Autodesk Fusion 360 part; units mm, degrees
sketch "Sketch1" plane through (0, 0, 0) normal (1, 0, 0) x (0, 1, 0)
  line L0 (0, 0) -> (27, 0)
  line L1 (27, 0) -> (27, 16)
  line L2 (27, 16) -> (0, 16)
  line L3 (0, 16) -> (0, 0)
  line L4 (0, 9.5) -> (6, 9.5) construction
  line L5 (6, 9.5) -> (6, 16) construction
  circle A0 centre (6, 9.5) radius 3
  line L6 (6, 9.5) -> (21, 9.5)
  circle A1 centre (21, 9.5) radius 3
  dimension "d1_4" = 16
  dimension "d2_4" = 27
  dimension "d3_4" = 6
  dimension "d4_4" = 6.5
  dimension "d5_2" = 6
  dimension "d6_1" = 15
  dimension "d7_2" = 6
extrude "Extrude1" add sketch "Sketch1" along normal blind 3 makes body 1
sketch "Sketch2" plane through (0, 0, 0) normal (-1, 0, 0) x (0, -1, 0)
  circle A0 centre (-21, 9.5) radius 3
  circle A1 centre (-6, 9.5) radius 3
  line L0 (0, 0) -> (0, 16)
  line L1 (0, 16) -> (-27, 16)
  line L2 (-27, 16) -> (-27, 0)
  line L3 (-27, 0) -> (0, 0)
  line L4 (0, 0) -> (-27, 0)
  line L5 (-27, 0) -> (-27, 3)
  line L6 (-27, 3) -> (0, 3)
  line L7 (0, 3) -> (0, 0)
  dimension "d10_1" = 3
extrude "Extrude2" add sketch "Sketch2" along normal blind 13 contours L0 L2 L3 L4 L5 L6 L7 bodies 1
ref_plane "WorkPlane1" through (-6.5, 13.5, 1.5) normal (-1, 0, 0) x (0, 0, 1)
mirror "Mirror1" about plane through (-6.5, 13.5, 1.5) normal (-1, 0, 0) of "Extrude1" makes body 2
combine "Combine1" operation add target body 1 tool bodies 2
sketch "Sketch3" plane through (0, 27, 0) normal (0, 1, 0) x (-1, 0, 0)
  line L0 (0, 3) -> (0, 16)
  line L1 (0, 16) -> (-3, 16)
  line L2 (-3, 16) -> (-3, 0)
  line L3 (-3, 0) -> (16, 0)
  line L4 (16, 0) -> (16, 16)
  line L5 (16, 16) -> (13, 16)
  line L6 (13, 16) -> (13, 3)
  line L7 (13, 3) -> (0, 3)
  line L8 (-3, 16) -> (16, 16)
  line L9 (16, 16) -> (16, 0)
  line L10 (16, 0) -> (-3, 0)
  line L11 (-3, 0) -> (-3, 16)
extrude "Extrude3" add sketch "Sketch3" along normal blind 3 bodies 1
sketch "Sketch4" plane through (0, 0, 0) normal (0, 0, -1) x (1, 0, 0)
  line L0 (3, -30) -> (3, 0)
  line L1 (3, 0) -> (-16, 0)
  line L2 (-16, 0) -> (-16, -30)
  line L3 (-16, -30) -> (3, -30)
  line L4 (-6.5, -30) -> (-6.5, -33) construction
  line L5 (7.5, -33) -> (-20.5, -33) construction
  line L6 (-20.5, -33) -> (-20.5, -61)
  line L7 (-20.5, -61) -> (7.5, -61)
  line L8 (7.5, -61) -> (7.5, -33)
  line L9 (-16, -30) -> (-20.5, -33)
  line L10 (3, -30) -> (7.5, -33)
  circle A0 centre (-6.5, -47) radius 11.5
  line L11 (7.5, -33) -> (-20.5, -61) construction
  line L12 (7.5, -61) -> (-20.5, -33) construction
  dimension "d23" = 28
  dimension "d24" = 28
  dimension "d25" = 3
  dimension "d28" = 23
extrude "Extrude4" add sketch "Sketch4" against normal blind 3 contours L3 L6 L7 L8 L9 L10 bodies 1
sketch "Sketch5" plane through (0, 0, 0) normal (0, 0, -1) x (1, 0, 0)
  circle A0 centre (-6.5, -47) radius 11.5
  line L0 (3, -30) -> (3, 0)
  line L1 (3, 0) -> (-16, 0)
  line L2 (-16, 0) -> (-16, -30)
  line L3 (-16, -30) -> (-20.5, -33)
  line L4 (-20.5, -33) -> (-20.5, -61)
  line L5 (-20.5, -61) -> (7.5, -61)
  line L6 (7.5, -61) -> (7.5, -33)
  line L7 (7.5, -33) -> (3, -30)
  line L8 (7.5, -61) -> (-20.5, -61)
  line L9 (-20.5, -61) -> (-20.5, -33)
  line L10 (-20.5, -33) -> (7.5, -33)
  line L11 (7.5, -33) -> (7.5, -61)
  line L12 (5, -58.5) -> (-18, -58.5) construction
  line L13 (-18, -58.5) -> (-18, -35.5) construction
  line L14 (-18, -35.5) -> (5, -35.5) construction
  line L15 (5, -35.5) -> (5, -58.5) construction
  circle A1 centre (5, -58.5) radius 1.5
  circle A2 centre (-18, -58.5) radius 1.5
  circle A3 centre (5, -35.5) radius 1.5
  circle A4 centre (-18, -35.5) radius 1.5
  dimension "d29" = 23
  dimension "d30" = 23
  dimension "d31" = 2.5
  dimension "d32" = 2.5
  dimension "d33" = 2.5
  dimension "d34" = 2.5
  dimension "d35" = 3
  dimension "d36" = 3
  dimension "d37" = 3
  dimension "d38" = 3
extrude "Extrude5" cut sketch "Sketch5" against normal up to surface (3 mm away) contours A1 | A2 | A3 | A4 bodies 1
sketch "Sketch10" plane through (0, 0, 3) normal (0, 0, 1) x (-1, 0, 0)
  circle A0 centre (-5, -35.5) radius 1.5
  circle A1 centre (18, -35.5) radius 1.5
  circle A2 centre (-5, -58.5) radius 1.5
  circle A3 centre (18, -58.5) radius 1.5
  circle A4 centre (6.5, -47) radius 11.5
  line L0 (20.5, -33) -> (16, -30)
  line L1 (16, -30) -> (-3, -30)
  line L2 (-3, -30) -> (-7.5, -33)
  line L3 (-7.5, -33) -> (-7.5, -61)
  line L4 (-7.5, -61) -> (20.5, -61)
  line L5 (20.5, -61) -> (20.5, -33)
  line L6 (-7.5, -61) -> (-10.5, -61)
  line L7 (-10.5, -61) -> (-10.5, -33)
  line L8 (-3, -26.5806) -> (-10.5, -31.5806)
  line L9 (-10.5, -31.5806) -> (-10.5, -61)
  line L10 (-3, 0) -> (-3, -30)
  line L11 (-7.5, -61) -> (-7.5, -61)
  dimension "d91" = 3
extrude "Extrude8" add sketch "Sketch10" along normal up to surface (13 mm away) and the other way up to surface (3 mm away) contours L2 L3 L6 L7 L8 L9 L10 bodies 1
mirror "Mirror3" about plane through (-6.5, 13.5, 1.5) normal (-1, 0, 0) of "Extrude8"
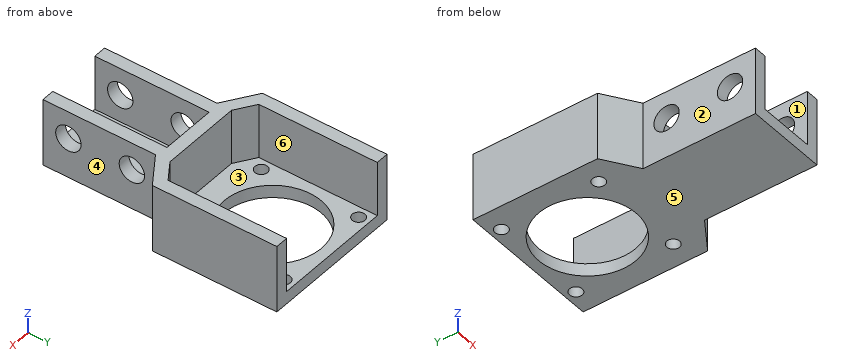
Check sheet for the modelled part. Datum: model origin and axes. Units: mm. Face numbers are marked on the shaded views. A direction names the side the tool comes from. Coordinates: 2 decimals unless noted, no trailing zeros. Write each loop counter-clockwise with the first axis right and the second up, starting at its lowest first coordinate (ties: lowest second). Pieces come first, ordered by that corner, then holes.
Item 1: Depth check by flat-ended pin: pin 1 Ø6.5 at (x, z) = (-4, 9) entering from -Y; pin 2 Ø10 at (x, y) = (-10, 36.5) entering from +Z; pin 3 Ø5 at (y, z) = (17.5, 7) entering from +X. Enter the tip coordinate at first touch or a pass-through.
Numbers:
pin 1: stops at y = 27
pin 2: stops at z = 3
pin 3: stops at x = 3
Item 2: Access from +Z, -Z, +X, -X, +Y, -Y to the whole of each face (thin tool, end or side, straight path). Record for the marked faces 1, 2 and 3.
Numbers:
face 1: +Z, -Y
face 2: +Z, -Z, -X, -Y
face 3: +Z, +Y
Item 3: Cross-section at C-C on y = 47. Record the boundary of the cut face in (x, z), then the cut area to 3 significant figures.
Numbers:
outline: (-23.5, 0) - (-18, 0) - (-18, 3) - (-20.5, 3) - (-20.5, 16) - (-23.5, 16) - close; (5, 0) - (10.5, 0) - (10.5, 16) - (7.5, 16) - (7.5, 3) - (5, 3) - close
area: 111 mm2
Item 4: Scan lines: probe 1 along X at (y, z) = (53, 15); probe 2 along Z at (x, y) = (1.25, 21); probe 3 along X at (y, z) = (20, 3.75). Record each from-to range of solid material in increasing order.
Numbers:
probe 1: x = -23.5 to -20.5, 7.5 to 10.5
probe 2: z = 0 to 6.5, 12.5 to 16
probe 3: x = -16 to -13, 0 to 3
Item 5: Cross-section at D-D on z = 9.5. Count the separate pieces of the cut face and the enclosed holes in it, then the cut area to 3 significant figures.
Numbers:
separate pieces: 5
enclosed holes: 0
area: 360 mm2
Item 6: Cross-section at B-B on x = -6. Record the boundary of the cut face in (y, z).
Numbers:
outline: (0, 0) - (35.51, 0) - (35.51, 3) - (30, 3) - (30, 16) - (27, 16) - (27, 3) - (0, 3) - close; (58.49, 0) - (61, 0) - (61, 3) - (58.49, 3) - close
Item 7: Cross-section at A-A on y = 6. Record the boundary of the cut face in (x, z).
Numbers:
outline: (-16, 0) - (3, 0) - (3, 6.5) - (0, 6.5) - (0, 3) - (-13, 3) - (-13, 6.5) - (-16, 6.5) - close; (-16, 12.5) - (-13, 12.5) - (-13, 16) - (-16, 16) - close; (0, 12.5) - (3, 12.5) - (3, 16) - (0, 16) - close
Item 8: Mould release check, pull along X, two halves, no side actions. Record for the marked faces 4, 5 and 6: released by +X, released by -X, zero draft, split by the parting line, or undercut.
Numbers:
face 4: released by +X
face 5: zero draft
face 6: undercut
